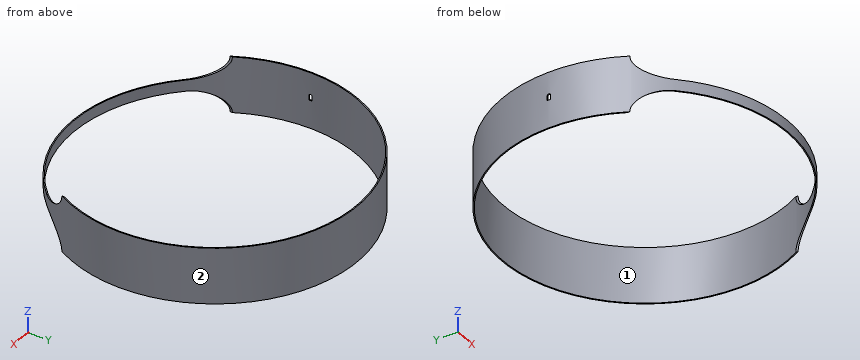
from build123d import *

# Parameters (mm, degrees)
SKETCH_3_R          = 64
SKETCH_3_R_2        = 63.5
EXTRUDE_2_DEPTH     = 25
CUT_EXTRUDE_2_DEPTH = 200
CUT_EXTRUDE_3_DEPTH = 200


with BuildPart() as part:
    # 草图3 → 凸台-拉伸2 (new body)
    with BuildSketch(Plane.XY):
        Circle(SKETCH_3_R)
        Circle(SKETCH_3_R_2, mode=Mode.SUBTRACT)
    extrude(amount=EXTRUDE_2_DEPTH)

    # 草图4 → 切除-拉伸2 (cut)
    with BuildSketch(Plane(origin=(0, 0, 0), x_dir=(1, 0, 0), z_dir=(0, 1, 0))):
        with BuildLine():
            Line((-46, -10), (46, -10))
            ThreePointArc((46, -10), (53.071067812, -7.071067812), (56, 0))
            Line((56, 0), (-56, 0))
            ThreePointArc((-56, 0), (-53.071067812, -7.071067812), (-46, -10))
        make_face()
        with BuildLine():
            Line((-46, -15), (46, -15))
            ThreePointArc((46, -15), (53.071067812, -17.928932188), (56, -25))
            Line((56, -25), (-56, -25))
            ThreePointArc((-56, -25), (-53.071067812, -17.928932188), (-46, -15))
        make_face()
    extrude(amount=-CUT_EXTRUDE_2_DEPTH, mode=Mode.SUBTRACT)

    # 草图6 → 切除-拉伸3 (cut)
    with BuildSketch(Plane(origin=(0, 0, 0), x_dir=(0, 0, -1), z_dir=(1, 0, 0))):
        with BuildLine():
            Line((-12.5, -0.75), (-12.5, 0.75))
            Line((-12.5, 0.75), (-14.5, 0.75))
            ThreePointArc((-14.5, 0.75), (-15.25, 0), (-14.5, -0.75))
            Line((-14.5, -0.75), (-12.5, -0.75))
        make_face()
    extrude(amount=-CUT_EXTRUDE_3_DEPTH, mode=Mode.SUBTRACT)


solid = part.part
Model file for the job. Use its own axes, mm. Face numbers are marked on the shaded views. Coordinates: 2 decimals unless noted, no trailing zeros. Order: outer loops, then holes, each group sorted by start corner. A loop starts at its lowest first (then second) coordinate and runs counter-clockwise, first axis right, second up. Notation, with made-up numbers: M 47.5,59.5 L 96.5,59.5 A14 cw 96.5,63.5 Z; hole C 51,50.25 d4. An arc over 180 degrees is marked long. Return JSON: item names as keys, results as strings.
1. Saw through at B-B (y = 3). Give the cut face in (x, z).
Ans:
{"outline": "M -63.93,0 L -63.43,0 L -63.43,25 L -63.93,25 Z; M 63.43,0 L 63.93,0 L 63.93,25 L 63.43,25 Z"}
2. Drill centre lines: probe 1 along Y at (x, z) = (0, 14.75); probe 2 along X at (y, z) = (0, 15). Where is each one in solid material? Low to high.
Ans:
{"probe 1": "-64 to -63.5, 63.5 to 64", "probe 2": "63.5 to 64"}
3. Saw through at A-A (x = 0). Give the cut face in (y, z).
Ans:
{"outline": "M -64,10 L -63.5,10 L -63.5,15 L -64,15 Z; M 63.5,0 L 64,0 L 64,25 L 63.5,25 Z"}
4. Pull direction X, two halves, no side cores. Call the marked faces 1 and 2: +X half, -X half, draft (parallel to the pull), parting line (faces both ways), or undercut.
Ans:
{"face 1": "undercut", "face 2": "parting line"}
5. Flat gauge pins, fed straight in: pin 1 (2 mm diameter, centred on x = 42.5, z = 22, fed in from -Y); pin 2 (22 mm diameter, centred on x = -18.5, y = -59, fed in from +Z); pin 3 (8 mm diameter, centred on y = 28, z = 4, fed in from -X); pin 4 (10 mm diameter, centred on x = 9.5, y = -54, fed in from -Z). Where does each tip first touch, or does it go through?
Ans:
{"pin 1": "y = 46.26", "pin 2": "z = 15", "pin 3": "x = -59.33", "pin 4": "through"}
